Geometry: final body of the model. Coordinates: model frame, mm. Face numbers are marked on the shaded views. Round coordinates to 2 decimals unless told otherwise and drop trailing zeros. Order: outer loops, then holes, each group sorted by start corner. A loop starts at its lowest first (then second) coordinate and runs counter-clockwise, first axis right, second up. Notation, with made-up numbers: M -2.5,13.5 L 19.5,13.5 A13 ccw 19.5,35.5 Z; hole C 10.5,-26.75 d4. An arc over 180 degrees is marked long. Put each result on its own line as item: value. Start each with the question number.
1) Section B-B, the plane z = 31.5. Return loops of the section in (x, y).
2) Draft query along X for the marked faces 1, 2, 3 and 4. Return one class per face: pulls with the +X half, pulls with the -X half, needs draft (parallel to the pull), parting line crosses it, or undercut.
3) Section D-D, the plane z = 62.5. Return loops of the section in (x, y), then the cut area to 3 significant figures.
4) First-contact query: P1, Ø2, axis at y = -24.5, z = -4.5, coming from the -X side; P2, Ø2, axis at x = 52, y = -13.5, coming from the +Z side; P3, Ø5, axis at x = 31.5, y = -11, coming from the -Z side. Flat tips, straight axial feed; report the tip coordinate or a pass-through.
5) Material intervals for probe 1 along Z at (x, y) = (-99, -18); probe 2 along Z at (x, y) = (-89.5, -35); probe 3 along X at (y, z) = (-34.5, 19), sorted ascending. Write a range as [from, to].
6) Section A-A, the plane x = -85.5. Return loops of the section in (y, z), then the cut area to 3 significant figures.
7) Section C-C, the plane y = -23.5. Return loops of the section in (x, z).
from build123d import *

# Parameters (mm, degrees)
F1_DEPTH = 50
F2_W     = 32.1948009557
F2_H     = 50
F3_DEPTH = 15.5
F4_R     = 25
F5_DEPTH = 50.001


with BuildPart() as f1:
    # F0 (on Front) → F1 (new body)
    with BuildSketch(Plane.XZ):
        with BuildLine():
            ThreePointArc((-39.5141846856, -29.3770225464), (-16.6691602535, -7.3325556277), (-8.2703797283, 23.2830310679))
            ThreePointArc((-8.2703797283, 23.2830310679), (-16.8774367266, 54.2469683115), (-40.2292267158, 76.3272931302))
            ThreePointArc((-40.2292267158, 76.3272931302), (-128.2690070017, 22.8771674096), (-39.5141846856, -29.3770225464))
        make_face()
        with BuildLine():
            ThreePointArc((-40.2292267158, 76.3272931302), (-16.8774367266, 54.2469683115), (-8.2703797283, 23.2830310679))
            ThreePointArc((-8.2703797283, 23.2830310679), (-16.6691602535, -7.3325556277), (-39.5141846856, -29.3770225464))
            Line((-39.5141846856, -29.3770225464), (45.1779214949, 0))
            ThreePointArc((45.1779214949, 0), (29.3226828607, 23.709159184), (49.4534202451, 43.9147582526))
            Line((49.4534202451, 43.9147582526), (-40.2292267158, 76.3272931302))
        make_face()
        with BuildLine():
            ThreePointArc((74.2167987014, 21.5288895412), (66.8052708694, 38.2198454046), (49.4534202451, 43.9147582526))
            ThreePointArc((49.4534202451, 43.9147582526), (29.3226828607, 23.709159184), (45.1779214949, 0))
            ThreePointArc((45.1779214949, 0), (65.1168968886, 3.454394567), (74.2167987014, 21.5288895412))
        make_face()
    extrude(amount=F1_DEPTH)

    # F2 (on face) → F3 (cut)
    with BuildSketch(Plane(origin=(19.7511057602, 0, 54.6495808388), x_dir=(0.9404629658, 0, -0.3398961752), z_dir=(0.3398961752, 0, 0.9404629658))):
        with Locations((-16.0974004779, -25)):
            Rectangle(F2_W, F2_H)
    extrude(amount=-F3_DEPTH, mode=Mode.SUBTRACT)

    # F4 (on face) → F5 (cut, through all)
    with BuildSketch(Plane.XZ.offset(50)):
        with Locations((-83.2891840334, 24.2245818774)):
            Circle(F4_R)
    extrude(amount=-F5_DEPTH, mode=Mode.SUBTRACT)


solid = f1.part
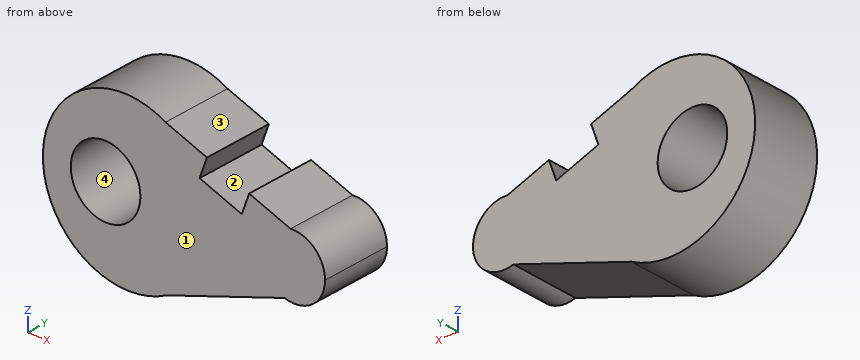
Result sheet:
1. outline: M -127.71,-50 L -107.21,-50 L -107.21,0 L -127.71,0 Z; M -59.37,-50 L 71.89,-50 L 71.89,0 L -59.37,0 Z
2. face 1: needs draft
2. face 2: undercut
2. face 3: pulls with the +X half
2. face 4: undercut
3. outline: M -113.68,-50 L -11.64,-50 L -11.64,0 L -113.68,0 Z
3. area: 5,100 mm2
4. P1: stops at x = -121.96
4. P2: stops at z = 44.03
4. P3: stops at z = -5.61
5. probe 1: z = [-28.25, 4.78], [43.67, 74.82]
5. probe 2: z = [-32.84, 0.01], [48.44, 79.4]
5. probe 3: x = [-128.12, -107.74], [-58.84, 74.07]
6. outline: M -50,-34.19 L 0,-34.19 L 0,-0.68 L -50,-0.68 Z; M -50,49.13 L 0,49.13 L 0,80.76 L -50,80.76 Z
6. area: 3,260 mm2
7. outline: M -40.23,76.33 A60 ccw long -39.51,-29.38 L 45.18,0 A22.5 ccw long 49.45,43.91 L 19.75,54.65 L 14.48,40.07 L -15.8,51.02 L -10.53,65.59 Z; hole C -83.29,24.22 d50
